```python
from build123d import *

# Parameters (mm, degrees)
EXTRUDE1_DEPTH = 10


with BuildPart() as part:
    # Sketch1 → Extrude1 (new body)
    with BuildSketch(Plane.XY):
        with BuildLine():
            Line((-3, 0), (-67, 0))
            ThreePointArc((-67, 0), (-69.121320344, -0.878679656), (-70, -3))
            Line((-70, -3), (-70, -6))
            ThreePointArc((-70, -6), (-70.878679656, -8.121320344), (-73, -9))
            Line((-73, -9), (-418.5, -9))
            ThreePointArc((-418.5, -9), (-420.621320344, -9.878679656), (-421.5, -12))
            Line((-421.5, -12), (-421.5, -92))
            ThreePointArc((-421.5, -92), (-420.621320344, -94.121320344), (-418.5, -95))
            Line((-418.5, -95), (-254.5, -95))
            ThreePointArc((-254.5, -95), (-252.378679656, -94.121320344), (-251.5, -92))
            Line((-251.5, -92), (-251.5, -68))
            ThreePointArc((-251.5, -68), (-248.571067812, -60.928932188), (-241.5, -58))
            Line((-241.5, -58), (-77, -58))
            ThreePointArc((-77, -58), (-73.464466094, -59.464466094), (-72, -63))
            Line((-72, -63), (-72, -92))
            ThreePointArc((-72, -92), (-71.121320344, -94.121320344), (-69, -95))
            Line((-69, -95), (-3, -95))
            ThreePointArc((-3, -95), (-0.878679656, -94.121320344), (0, -92))
            Line((0, -92), (0, -3))
            ThreePointArc((0, -3), (-0.878679656, -0.878679656), (-3, 0))
        make_face()
        with BuildLine():
            Line((-403.5, -74.75), (-400, -74.75))
            ThreePointArc((-400, -74.75), (-392.75, -67.5), (-400, -60.25))
            Line((-400, -60.25), (-403.5, -60.25))
            ThreePointArc((-403.5, -60.25), (-410.75, -67.5), (-403.5, -74.75))
        make_face(mode=Mode.SUBTRACT)
        with BuildLine():
            Line((-403.5, -34.75), (-400, -34.75))
            ThreePointArc((-400, -34.75), (-392.75, -27.5), (-400, -20.25))
            Line((-400, -20.25), (-403.5, -20.25))
            ThreePointArc((-403.5, -20.25), (-410.75, -27.5), (-403.5, -34.75))
        make_face(mode=Mode.SUBTRACT)
    extrude(amount=EXTRUDE1_DEPTH)


solid = part.part
```
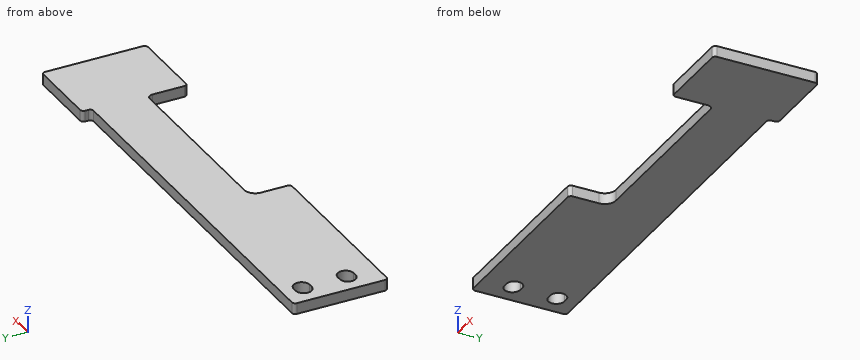
Here's how the part is built. I have some questions about the finished solid (model axes, mm). Round coordinates to 2 decimals unless told otherwise and drop trailing zeros. Order: outer loops, then holes, each group sorted by start corner. A loop starts at its lowest first (then second) coordinate and runs counter-clockwise, first axis right, second up. Notation, with made-up numbers: M 33,11.25 L 56,11.25 A14 cw 56,29.25 Z; hole C 75.5,35 d4. An arc over 180 degrees is marked long. Use CSV: the item, a comma, the result in double quotes.
1) I want a section at B-B (z = 3). List the corners of the cut face in (x, y) for me, then the cut area to 3 significant figures.
Taken from the geometry:
outline,"M -421.5,-92 A3 ccw -418.5,-95 L -254.5,-95 A3 ccw -251.5,-92 L -251.5,-68 A10 cw -241.5,-58 L -77,-58 A5 cw -72,-63 L -72,-92 A3 ccw -69,-95 L -3,-95 A3 ccw 0,-92 L 0,-3 A3 ccw -3,0 L -67,0 A3 ccw -70,-3 L -70,-6 A3 cw -73,-9 L -418.5,-9 A3 ccw -421.5,-12 Z; hole M -403.5,-74.75 L -400,-74.75 A7.25 ccw -400,-60.25 L -403.5,-60.25 A7.25 ccw Z; hole M -403.5,-34.75 L -400,-34.75 A7.25 ccw -400,-20.25 L -403.5,-20.25 A7.25 ccw Z"
area,"29,800 mm^2"
2) I need wall thicknesses on line 1 along Y through (x, z) = (-402.5, 3.25); line 2 along X through (y, z) = (-68.5, 4.25); line 3 along X through (y, z) = (-70.5, 9.5). Which ranges of each line are inside material? Lowest first, please. Write a range as [from, to].
Taken from the geometry:
line 1,"[-95, -74.75], [-60.25, -34.75], [-20.25, -9]"
line 2,"[-421.5, -410.68], [-392.82, -251.5], [-72, 0]"
line 3,"[-421.5, -410.1], [-393.4, -251.5], [-72, 0]"
3) I want a section at D-D (x = -303.5). List the corners of the cut face in (y, z) for me, then the cut area to 3 significant figures.
Taken from the geometry:
outline,"M -95,0 L -9,0 L -9,10 L -95,10 Z"
area,"860 mm^2"
4) I want a section at A-A (y = -27.5). List the corners of the cut face in (x, z) for me, then the cut area to 4 significant figures.
Taken from the geometry:
outline,"M -421.5,0 L -410.75,0 L -410.75,10 L -421.5,10 Z; M -392.75,0 L 0,0 L 0,10 L -392.75,10 Z"
area,"4,035 mm^2"
5) I'm going to push flat-ended pins straight in: P1, Ø5, axis at x = -218.5, z = 3.5, coming from the -Y side; P2, Ø3, axis at x = -401, z = 7, coming from the +Y side; P3, Ø1.5, axis at y = -4, z = 3, coming from the -X side. Where does each tip first touch, or does it pass through?
Taken from the geometry:
P1,"y = -58"
P2,"y = -9"
P3,"x = -70"
6) I want a section at C-C (x = -155.5). List the corners of the cut face in (y, z) for me.
Taken from the geometry:
outline,"M -58,0 L -9,0 L -9,10 L -58,10 Z"
